```python
from build123d import *

# Parameters (mm, degrees)
F2_R     = 3.75
F2_R_2   = 4.85
F3_DEPTH = 30.001
F4_SIZE  = 2


with BuildPart() as f1:
    # F0 (on Front) → F1 (revolve)
    with BuildSketch(Plane.XZ):
        Polygon((16, 15), (0, 15), (0, -15), (16, -15), (16, -11), (16.5, -10.5), (16.5, -8.5), (16, -8), (16, -4.666667), (16.5, -4.166667), (16.5, -2.166667), (16, -1.666667), (16, 1.666667), (16.5, 2.166667), (16.5, 4.166667), (16, 4.666667), (16, 8), (16.5, 8.5), (16.5, 10.5), (16, 11), align=None)
    revolve(axis=Axis((0, 0, 0), (0, 0, -1)))

    # F2 (on face) → F3 (cut, through all)
    with BuildSketch(Plane.XY.offset(15)):
        with Locations((-6.25, 0)):
            Circle(F2_R)
        with Locations((6.25, 0)):
            Circle(F2_R_2)
    extrude(amount=-F3_DEPTH, mode=Mode.SUBTRACT)

    # F4
    f4_edges = [f1.edges().sort_by_distance(p)[0] for p in [
        (-16, 0, -15),
    ]]
    chamfer(f4_edges, length=F4_SIZE)


solid = f1.part
```
Geometry: final body of the model. Coordinates: model frame, mm. A direction names the side the tool comes from. Give positions to 0.01 mm unless a question says otherwise; leave off trailing zeros. Loops run counter-clockwise (first coordinate to the right, second up) from the corner with the lowest first, then second, coordinate; pieces in that order, holes last. Notation, with made-up numbers: (23, -3) -> (33, -3) arc R21 ccw to (33, 11) -> close; hole circle Ø4 at (52.5, 64.5). An arc over 180 degrees is marked (long way). Use one line per item in the form item = value.
Item 1: Line query: probe 1 along X at (y, z) = (-2, 2.75); probe 2 along X at (y, z) = (1, -1.25); probe 3 along Z at (x, y) = (6, 15). Output: solid intervals per line, ascending.
A:
probe_1 = -16.38 to -9.42, -3.08 to 1.83, 10.67 to 16.38
probe_2 = -15.97 to -9.86, -2.64 to 1.5, 11 to 15.97
probe_3 = -10.84 to -8.16, -4.51 to -1.82, 1.82 to 4.51, 8.16 to 10.84
Item 2: Draft query along Z for faces 1 (the face through (-3.062, 13.789, -14.875)), 2 (the face through (-3.47, 15.62, 13.03)), 3 (the face through (-3.47, 15.62, 6.36)), 4 (the face through (0, 0, 15)). Return one class per face: pulls with the +Z half, pulls with the -Z half, needs draft (parallel to the pull), parting line crosses it, or undercut.
A:
face_1 = pulls with the -Z half
face_2 = needs draft
face_3 = undercut
face_4 = pulls with the +Z half
Item 3: Access query for faces 5 (the face through (-3.47, 15.62, -6.31)), 6 (the face through (15.24, 6.32, 9.51)). Directions: +Z, -Z, +X, -X, +Y, -Y. A direction counts if a zero-diameter tool reaches every point of the face in a straight line with its end or side. Return the directions, or none.
A:
face_5 = none
face_6 = +Z, -Z
Item 4: Pin query (flat end, axial travel): P1, Ø4, axis at x = -3.5, z = -11.5, coming from the +Y side (3 decimals); P2, Ø4, axis at y = 11, z = 4, coming from the +X side; P3, Ø5, axis at x = -7.5, z = 0, coming from the +Y side; P4, Ø10, axis at x = -0.5, z = 7, coming from the +Y side. Return the tip coordinate at first contact, or that it passes through.
A:
P1 = 16.405
P2 = 13.83
P3 = 15.27
P4 = 16.5
Item 5: Section query B-B on z = -6. Output: boundary loops of the cut face in (x, y), and give its area (3 significant figures).
A:
outline = circle Ø32 at (0, 0); hole circle Ø7.5 at (-6.25, 0); hole circle Ø9.7 at (6.25, 0)
area = 686 mm^2
Item 6: Section query A-A on y = 0. Give the number of separate pieces and of enclosed holes in the cut face, and give its area (3 significant figures).
A:
separate_pieces = 3
enclosed_holes = 0
area = 450 mm^2
